Geometry check sheet. Reference: the model listing, model coordinates, mm. A direction names the side the tool comes from. Give positions to 0.01 mm unless a question says otherwise; leave off trailing zeros. Loops run counter-clockwise (first coordinate to the right, second up) from the corner with the lowest first, then second, coordinate; pieces in that order, holes last. Notation, with made-up numbers: (81.5, 32) -> (86.5, 32) arc R20 cw to (86.5, 42) -> close; hole circle Ø1 at (-1.5, 1). An arc over 180 degrees is marked (long way). Write item = value, one per line. Start each with the question number.
```python
from build123d import *

# Parameters (mm, degrees)
F2_W     = 50.5212787539
F2_H     = 4.6267285943
F4_W     = 50.5212787539
F4_H     = 2.9346304946
F5_DEPTH = 20.066
F6_DEPTH = 25.4
F4_H_2   = 2.5909789344
F7_DEPTH = 20.32


with BuildPart() as f3:
    # F3: sweep along a path in F0
    with BuildLine(Plane.YZ) as f3_path:
        Line((-55.8239743114, -18.6951477081), (-40.2851480178, -18.6951477081))
        ThreePointArc((-40.2851480178, -18.6951477081), (-37.0180999924, -17.7902277993), (-34.682206865, -15.3333830466))
        Line((-34.682206865, -15.3333830466), (-9.579990698, 31.7332713683))
        ThreePointArc((-9.579990698, 31.7332713683), (-7.2440975706, 34.190116121), (-3.9770495452, 35.0950360298))
        Line((-3.9770495452, 35.0950360298), (89.1171097755, 35.0950360298))
    # F2 (on offset) → F3 (sweep)
    with BuildSketch(Plane.XZ.offset(55.88)):
        with Locations((-14.3274748698, -19.7674240917)):
            Rectangle(F2_W, F2_H)
    sweep(path=f3_path.line)

    # F4 (on face) → F5 (join)
    with BuildSketch(Plane(origin=(0, 0, 31.709395349), x_dir=(1, 0, 0), z_dir=(0, 0, -1))):
        with Locations((-14.3274748698, -7.4532397557)):
            Rectangle(F4_W, F4_H)
    extrude(amount=F5_DEPTH)

    # F4 (on face) → F6 (join)
    with BuildSketch(Plane(origin=(0, 0, 31.709395349), x_dir=(1, 0, 0), z_dir=(0, 0, -1))):
        with Locations((-14.3274748698, -7.4532397557)):
            Rectangle(F4_W, F4_H)
        Polygon((10.9331645072, -17.0301664621), (10.9331645072, -14.2893027514), (-39.5881142467, -14.9312503636), (-39.5881142467, -17.0301664621), align=None)
    extrude(amount=F6_DEPTH)

    # F4 (on face) → F7 (join)
    with BuildSketch(Plane(origin=(0, 0, 31.709395349), x_dir=(1, 0, 0), z_dir=(0, 0, -1))):
        with Locations((-14.3274748698, -24.7733006254)):
            Rectangle(F4_W, F4_H_2)
    extrude(amount=F7_DEPTH)


solid = f3.part
```
1) Section check C-C (y = 49). Enter the section's corners in (x, z).
2) Section check D-D (z = 8). Enter the section's corners in (x, y).
3) Tool access check on faces 4 (the flat face through (-15, 7, 6.309)), 5 (the flat face through (-14, -48, -17.454)), 6 (the cylindrical face through (-13.974, -5.569, 31.246)), 7 (the flat face through (-14, -55.88, -20)). Record the directions out of +Z, -Z, +X, -X, +Y, -Y that give a thin tool (end or side, any length) a straight path to the whole face; none if there is none.
4) Draft check along Y on faces 1 (the cylindrical face through (-14.681, -7.98, 35.195)), 2 (the flat face through (-15, 12, 31.709)), 3 (the flat face through (-39.588, 6.2, 20.2)). Enter one of: released by +Y, released by -Y, zero draft, split by the parting line, or undercut.
5) Thickness scan on line 1 (Y direction, x = -31, z = 14); line 2 (Y direction, x = 0, z = 24.5); line 3 (Y direction, x = -32.5, z = 6.5). Record the ranges inside material, lowest first.
6) Section check B-B (x = 3.5). Enter the section's corners in (y, z), plus the area to 3 significant figures.
7) Section check A-A (z = 26). Enter the section's corners in (x, y), plus the area to 3 significant figures.
8) Depth check by flat-ended pin: pin 1 Ø12.5 at (x, z) = (-6.5, 20.5) entering from -Y; pin 2 Ø17 at (x, y) = (-13.5, -47) entering from +Z; pin 3 Ø4 at (x, y) = (-13, -37) entering from -Z. Enter the tip coordinate at first touch or a pass-through.
Check result:
q1.outline = (-39.59, 31.71) -> (10.93, 31.71) -> (10.93, 36.34) -> (-39.59, 36.34) -> close
q2.outline = (-39.59, -23.64) -> (10.93, -23.64) -> (10.93, -18.4) -> (-39.59, -18.4) -> close; (-39.59, 5.99) -> (10.93, 5.99) -> (10.93, 8.92) -> (-39.59, 8.92) -> close; (-39.59, 14.93) -> (10.93, 14.29) -> (10.93, 17.03) -> (-39.59, 17.03) -> close
q3.face_4 = -Z, +X, -X, +Y
q3.face_5 = +Z, +X, -X, -Y
q3.face_6 = -Z, +X, -X
q3.face_7 = +Z, -Z, +X, -X, -Y
q4.face_1 = released by -Y
q4.face_2 = undercut
q4.face_3 = zero draft
q5.line_1 = -20.44 to -15.2, 5.99 to 8.92, 14.82 to 17.03, 23.48 to 26.07
q5.line_2 = -14.84 to -9.6, 5.99 to 8.92, 14.43 to 17.03, 23.48 to 26.07
q5.line_3 = -24.44 to -19.2, 5.99 to 8.92, 14.84 to 17.03
q6.outline = (-55.88, -22.08) -> (-40.34, -22.08) arc R9.74 ccw to (-31.72, -16.98) -> (-6.62, 30.09) arc R2.96 cw to (-4.03, 31.71) -> (5.99, 31.71) -> (5.99, 6.31) -> (8.92, 6.31) -> (8.92, 31.71) -> (14.38, 31.71) -> (14.38, 6.31) -> (17.03, 6.31) -> (17.03, 31.71) -> (23.48, 31.71) -> (23.48, 11.39) -> (26.07, 11.39) -> (26.07, 31.71) -> (89.06, 31.71) -> (89.06, 36.34) -> (-4.03, 36.34) arc R7.59 ccw to (-10.7, 32.27) -> (-35.8, -14.8) arc R5.11 cw to (-40.34, -17.45) -> (-55.88, -17.45) -> close
q6.area = 1,010 mm2
q7.outline = (-39.59, -14.04) -> (10.93, -14.04) -> (10.93, -8.8) -> (-39.59, -8.8) -> close; (-39.59, 5.99) -> (10.93, 5.99) -> (10.93, 8.92) -> (-39.59, 8.92) -> close; (-39.59, 14.93) -> (10.93, 14.29) -> (10.93, 17.03) -> (-39.59, 17.03) -> close; (-39.59, 23.48) -> (10.93, 23.48) -> (10.93, 26.07) -> (-39.59, 26.07) -> close
q7.area = 666 mm2
q8.pin_1 = -20.31
q8.pin_2 = -17.13
q8.pin_3 = -22
